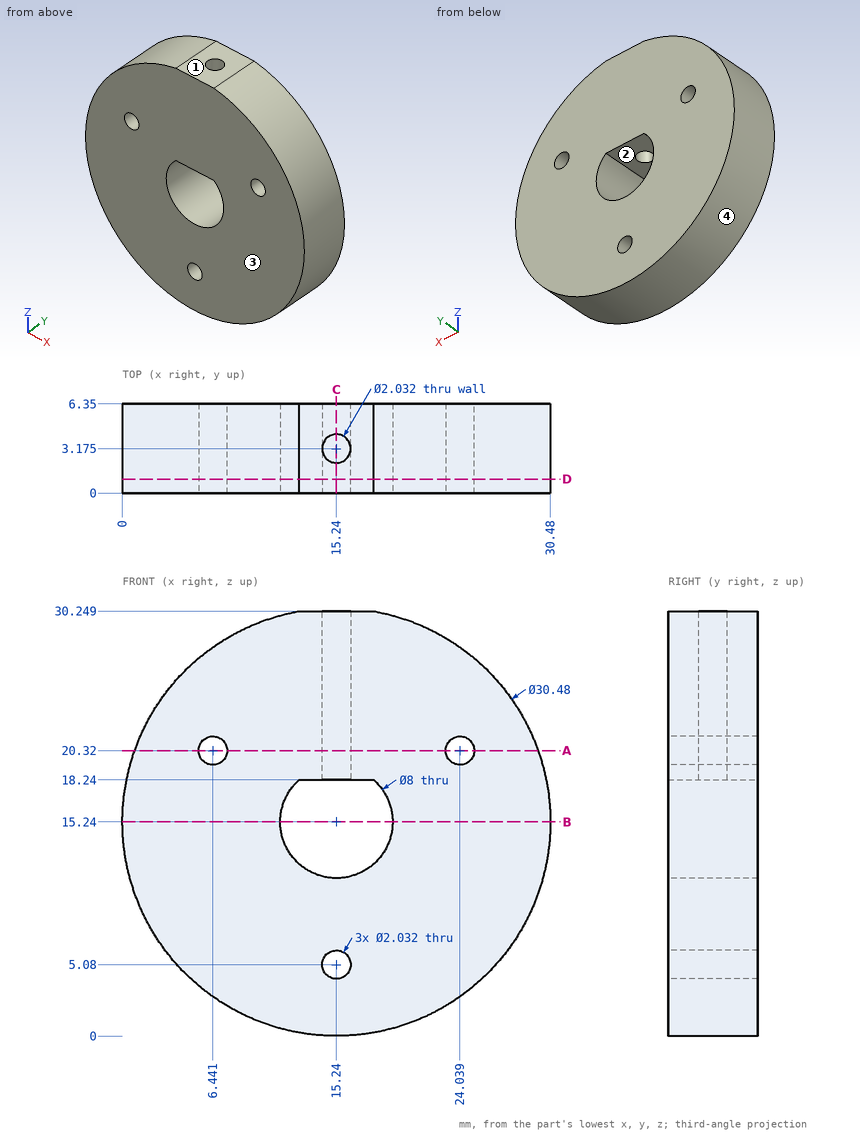
Source: three-view drawing plus pictorial views. Frame: mm from the lowest corner of the part. Round coordinates to 2 decimals unless told otherwise and drop trailing zeros. Loops run counter-clockwise (first coordinate to the right, second up) from the corner with the lowest first, then second, coordinate; pieces in that order, holes last.
1. Section query A-A on z = 20.32. Give the number of separate pieces and of enclosed holes in the cut face.
2. Contact query for flat-ended pins moving along their axis: pin 1 (1 mm diameter, centred on y = 4, z = 16.5, fed in from -X); pin 2 (3 mm diameter, centred on y = 5, z = 26, fed in from -X) (1 decimal). Output: stop coordinate, or through.
3. Ray query, L1, parallel to X at y = 1.5, z = 15.24; L2, parallel to X at y = 1.5, z = 20.5; L3, parallel to Z at x = 14, y = 2.75. Return the intervals inside material, ascending.
4. Mould query, pull axis Z, two halves, no side actions, for the marked faces 1, 2, 3 and 4. Classes: released by +Z, released by -Z, zero draft, split by the parting line, or undercut.
5. Section query B-B on z = 15.24. Output: boundary loops of the cut face in (x, y).
6. Section query C-C on x = 15.24. Output: boundary loops of the cut face in (y, z).
7. Section query D-D on y = 1. Output: boundary loops of the cut face in (x, z) (1 decimal).
Answers below:
1. separate pieces: 3
1. enclosed holes: 1
2. pin 1: stops at x = 0.02
2. pin 2: stops at x = 3.1
3. L1: x = 0 to 11.24, 19.24 to 30.48
3. L2: x = 0.94 to 5.44, 7.44 to 23.04, 25.04 to 29.54
3. L3: z = 0.05 to 11.44, 18.24 to 30.25
4. face 1: released by +Z
4. face 2: undercut
4. face 3: zero draft
4. face 4: split by the parting line
5. outline: (0, 0) - (11.24, 0) - (11.24, 6.35) - (0, 6.35) - close; (19.24, 0) - (30.48, 0) - (30.48, 6.35) - (19.24, 6.35) - close
6. outline: (0, 0) - (6.35, 0) - (6.35, 4.06) - (0, 4.06) - close; (0, 6.1) - (6.35, 6.1) - (6.35, 11.24) - (0, 11.24) - close; (0, 18.24) - (2.16, 18.24) - (2.16, 30.25) - (0, 30.25) - close; (4.19, 18.24) - (6.35, 18.24) - (6.35, 30.25) - (4.19, 30.25) - close
7. outline: (12.6, 30.2) arc R15.2 ccw (long way) to (17.9, 30.2) - close; hole circle Ø2 at (6.4, 20.3); hole (12.6, 18.2) arc R4 ccw (long way) to (17.9, 18.2) - close; hole circle Ø2 at (15.2, 5.1); hole circle Ø2 at (24, 20.3)
